```python
from build123d import *

# Parameters (mm, degrees)
BOSS_EXTRUDE1_DEPTH = 10
CUT_EXTRUDE1_DEPTH  = 82.115739792
SKETCH5_R           = 2.5
BOSS_EXTRUDE2_DEPTH = 10
FILLET1_R           = 0.5


with BuildPart() as part:
    # Sketch2 → Boss-Extrude1 (new body)
    with BuildSketch(Plane(origin=(0, 0, 0), x_dir=(1, 0, 0), z_dir=(0, 1, 0))):
        with BuildLine():
            Line((-19.893799085, 78), (0, 78))
            Line((0, 78), (0, 76))
            ThreePointArc((0, 76), (-2.121320344, 75.121320344), (-3, 73))
            Line((-3, 73), (-3, 63))
            ThreePointArc((-3, 63), (-2.121320344, 60.878679656), (0, 60))
            Line((0, 60), (0, 3))
            ThreePointArc((0, 3), (-2.121320344, 2.121320344), (-3, 0))
            Line((-3, 0), (-3, -10))
            ThreePointArc((-3, -10), (-2.121320344, -12.121320344), (0, -13))
            Line((0, -13), (0, -15))
            Line((0, -15), (-19.893799085, -15))
            Line((-19.893799085, -15), (-19.893799085, 78))
        make_face()
    boss_extrude1 = extrude(amount=BOSS_EXTRUDE1_DEPTH)

    # Mirror1: Boss-Extrude1 across Right Plane
    add(boss_extrude1.mirror(Plane(origin=(0, 0, 0), x_dir=(0, 0, -1), z_dir=(1, 0, 0))))

    # Sketch4 → Cut-Extrude1 (cut, through all)
    with BuildSketch(Plane(origin=(0, 0, 0), x_dir=(1, 0, 0), z_dir=(0, 1, 0))):
        with BuildLine():
            Line((-15, 15), (-15, 5))
            ThreePointArc((-15, 5), (-12, 2), (-9, 5))
            Line((-9, 5), (-9, 15))
            ThreePointArc((-9, 15), (-12, 18), (-15, 15))
        make_face()
        with BuildLine():
            Line((15, 48), (15, 58))
            ThreePointArc((15, 58), (12, 61), (9, 58))
            Line((9, 58), (9, 48))
            ThreePointArc((9, 48), (12, 45), (15, 48))
        make_face()
    extrude(amount=CUT_EXTRUDE1_DEPTH, mode=Mode.SUBTRACT)

    # Sketch5 → Boss-Extrude2 (add)
    with BuildSketch(Plane(origin=(0, 10, 0), x_dir=(1, 0, 0), z_dir=(0, 1, 0))):
        with Locations(Location((0, 31.5, 0), (0, 0, 270))):
            Circle(SKETCH5_R)
    extrude(amount=BOSS_EXTRUDE2_DEPTH)

    # Fillet1
    fillet1_edges = [part.edges().sort_by_distance(p)[0] for p in [
        (0, 10, -34),
    ]]
    fillet(fillet1_edges, radius=FILLET1_R)


solid = part.part
```
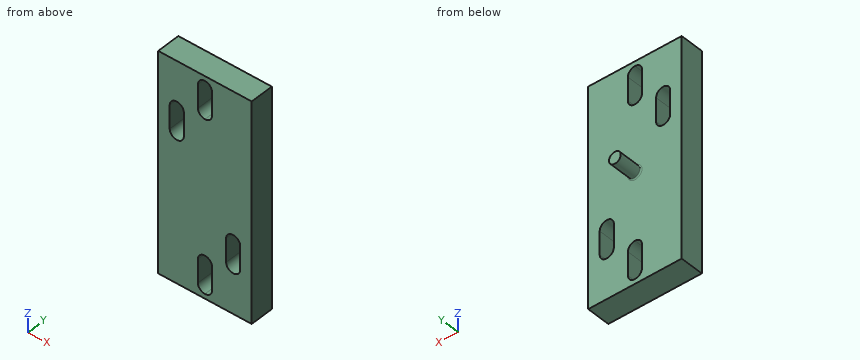
Design review of the part built by this model. Coordinates are the model's own, in mm. Coordinates: 2 decimals unless noted, no trailing zeros. Order: outer loops, then holes, each group sorted by start corner. A loop starts at its lowest first (then second) coordinate and runs counter-clockwise, first axis right, second up. Notation, with made-up numbers: M 15.5,18 L 58.5,18 A16 ccw 58.5,25 Z; hole C -16,39.25 d7. An arc over 180 degrees is marked long. Answer as a JSON object with one key per item and string values. Group by question number.
1) Add section A-A, the plane z = -67. Write out the cut boundary in (x, y).
2) Add section B-B, the plane x = -12. Write out the cut boundary in (y, z).
3) Add section C-C, the plane y = 8.5. Write out the cut boundary in (x, z).
4) Add section D-D, the plane z = -31.5. Write out the cut boundary in (x, y).
5) Wall thickness on L1, parallel to X at y = 1.75, z = -10; L2, parallel to X at y = 2, z = -49; L3, parallel to Y at x = 9, z = -40: over which ranges is each line inside the solid? List them lowest first.
Computed values:
{
 "1": {"outline": "M -19.89,0 L -3,0 L -3,10 L -19.89,10 Z; M 3,0 L 19.89,0 L 19.89,10 L 3,10 Z"},
 "2": {"outline": "M 0,-78 L 10,-78 L 10,-18 L 0,-18 Z; M 0,-2 L 10,-2 L 10,15 L 0,15 Z"},
 "3": {"outline": "M -19.89,-78 L 19.89,-78 L 19.89,15 L -19.89,15 Z; hole M -15,-15 A3 ccw -9,-15 L -9,-5 A3 ccw -15,-5 Z; hole M -3,-73 A3 ccw 3,-73 L 3,-63 A3 ccw -3,-63 Z; hole M -3,0 A3 ccw 3,0 L 3,10 A3 ccw -3,10 Z; hole M 9,-58 A3 ccw 15,-58 L 15,-48 A3 ccw 9,-48 Z"},
 "4": {"outline": "M -19.89,0 L 19.89,0 L 19.89,10 L 3,10 A0.5 cw 2.5,10.5 L 2.5,20 L -2.5,20 L -2.5,10.5 A0.5 cw -3,10 L -19.89,10 Z"},
 "5": {"L1": "x = -19.89 to -15, -9 to 19.89", "L2": "x = -19.89 to 9, 15 to 19.89", "L3": "y = 0 to 10"}
}
